Read the model definition and answer for the solid it produces. Units are mm, in the model's axes. A direction names the side the tool comes from. Coordinates: 2 decimals unless noted, no trailing zeros. Order: outer loops, then holes, each group sorted by start corner. A loop starts at its lowest first (then second) coordinate and runs counter-clockwise, first axis right, second up. Notation, with made-up numbers: (-19, -3.5) - (37, -3.5) arc R19 ccw to (37, 4.5) - close; hole circle Ø9 at (81, 10). An arc over 180 degrees is marked (long way). Write item = value, one per line.
from build123d import *

# Parameters (mm, degrees)
F0_R           = 18
F0_R_2         = 16
F1_DEPTH       = 7
F2_R           = 27.5
F2_R_2         = 16
F3_DEPTH       = 2
F4_R           = 18
F4_R_2         = 14
F5_DEPTH       = 2
F7_D           = 3.5
F7_CSINK_D     = 6
F7_CSINK_ANGLE = 90


with BuildPart() as f1:
    # F0 (on Top) → F1 (new body)
    with BuildSketch(Plane.XY):
        Circle(F0_R)
        Circle(F0_R_2, mode=Mode.SUBTRACT)
    extrude(amount=-F1_DEPTH)

    # F2 (on Top) → F3 (join)
    with BuildSketch(Plane.XY):
        Circle(F2_R)
        Circle(F2_R_2, mode=Mode.SUBTRACT)
    extrude(amount=F3_DEPTH)

    # F4 (on face) → F5 (join)
    with BuildSketch(Plane(origin=(0, 0, -7), x_dir=(1, 0, 0), z_dir=(0, 0, -1))):
        Circle(F4_R)
        Circle(F4_R_2, mode=Mode.SUBTRACT)
    extrude(amount=F5_DEPTH)

    # F7 (through all)
    with Locations(Plane.XY.offset(2)):
        with Locations((0, 22.5), (-19.485572, -11.25), (19.485572, -11.25)):
            CounterSinkHole(F7_D / 2, F7_CSINK_D / 2, counter_sink_angle=F7_CSINK_ANGLE)


solid = f1.part
1) For faces 4 (the face through (-21.155, -10.724, 0.37)), 5 (the face through (-3.47, -15.62, -2.56)), determine the directions among +Z, -Z, +X, -X, +Y, -Y from which every point of the face is accessible in a straight line to the end or side of a thin tool.
Returned:
face_4 = +Z, -Z
face_5 = +Z
2) Flat-ended cylindrical pins translate along their axes: pin 1 Ø1.5 at (x, z) = (-17, -3.5) entering from -Y; pin 2 Ø1.5 at (x, z) = (-4, -6) entering from -Y; pin 3 Ø1.5 at (y, z) = (-9, -6) entering from -X. Find the tip coordinate at first contact, or state that the pin passes through.
Returned:
pin_1 = -7.74
pin_2 = -17.7
pin_3 = -16
3) The part is cut by section A-A (y = 0). Determine the outline of the cut face in (x, z).
Returned:
outline = (-27.5, 0) - (-18, 0) - (-18, -9) - (-14, -9) - (-14, -7) - (-16, -7) - (-16, 2) - (-27.5, 2) - close; (14, -9) - (18, -9) - (18, 0) - (27.5, 0) - (27.5, 2) - (16, 2) - (16, -7) - (14, -7) - close
4) Determine the mould class of faces 1 (the face through (18, -6, 0)), 2 (the face through (17.816, -10.724, 0.37)), 3 (the face through (-2.343, -17.847, -4.437)) for opening direction Y: pulls with the +Y half, pulls with the -Y half, needs draft (parallel to the pull), parting line crosses it, or undercut.
Returned:
face_1 = needs draft
face_2 = undercut
face_3 = parting line crosses it
5) Straight lines are drawn through the part: line 1 along X through (y, z) = (0, -7.4); line 2 along Y through (x, z) = (0, -4.25); line 3 along X through (y, z) = (-11.25, 0.45). For each, find the intervals that lie inside material, in ascending order. Write a range as from..to.
Returned:
line_1 = -18..-14, 14..18
line_2 = -18..-16, 16..18
line_3 = -25.09..-21.24, -17.74..-11.38, 11.38..17.74, 21.24..25.09
6) The part is cut by section C-C (x = -8). Determine the outline of the cut face in (y, z), and give its area (3 significant figures).
Returned:
outline = (-26.31, 0) - (-16.12, 0) - (-16.12, -9) - (-11.49, -9) - (-11.49, -7) - (-13.86, -7) - (-13.86, 2) - (-26.31, 2) - close; (11.49, -9) - (16.12, -9) - (16.12, 0) - (26.31, 0) - (26.31, 2) - (13.86, 2) - (13.86, -7) - (11.49, -7) - close
area = 100 mm^2
7) The part is cut by section D-D (z = -3). Determine the outline of the cut face in (x, y), and give its area (3 significant figures).
Returned:
outline = circle Ø36 at (0, 0); hole circle Ø32 at (0, 0)
area = 214 mm^2
8) The part is cut by section B-B (x = 0). Determine the outline of the cut face in (y, z), and give its area (3 significant figures).
Returned:
outline = (-27.5, 0) - (-18, 0) - (-18, -9) - (-14, -9) - (-14, -7) - (-16, -7) - (-16, 2) - (-27.5, 2) - close; (14, -9) - (18, -9) - (18, 0) - (20.75, 0) - (20.75, 0.75) - (19.5, 2) - (16, 2) - (16, -7) - (14, -7) - close; (24.25, 0) - (27.5, 0) - (27.5, 2) - (25.5, 2) - (24.25, 0.75) - close
area = 81.4 mm^2
